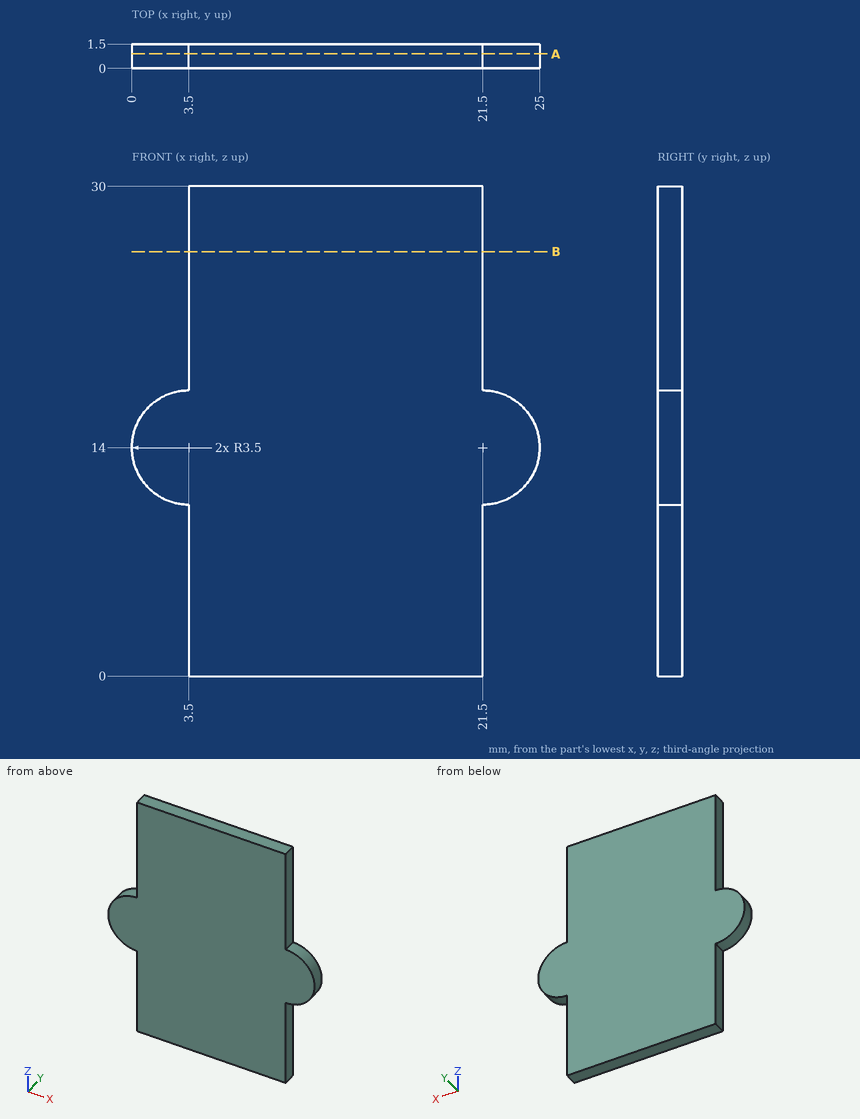
Geometry: see drawing. Coordinates: mm, zero at the bounding-box minimum. Round coordinates to 2 decimals unless told otherwise and drop trailing zeros. Write each loop counter-clockwise with the first axis right and the second up, starting at its lowest first coordinate (ties: lowest second). Pieces come first, ordered by that corner, then holes.
1) Cut plane B-B (z = 26). Return the cut outline in (x, y), then the cut area to 3 significant figures.
2) Contact query for a flat-ended pin moving along its axis: P1, Ø5, axis at x = 22.5, z = 22.5, coming from the -Y side. Output: stop coordinate, or through.
3) Cut plane A-A (y = 0.9). Return the cut outline in (x, z).
4) Ray query, L1, parallel to X at y = 1, z = 17.75; L2, parallel to X at y = 0.55, z = 11; L3, parallel to Z at x = 1, y = 1. Return the intervals inside material, ascending.
Geometry says:
1. outline: (3.5, 0) - (21.5, 0) - (21.5, 1.5) - (3.5, 1.5) - close
1. area: 27.0 mm2
2. P1: stops at y = 0
3. outline: (3.5, 0) - (21.5, 0) - (21.5, 10.5) arc R3.5 ccw to (21.5, 17.5) - (21.5, 30) - (3.5, 30) - (3.5, 17.5) arc R3.5 ccw to (3.5, 10.5) - close
4. L1: x = 3.5 to 21.5
4. L2: x = 1.7 to 23.3
4. L3: z = 11.55 to 16.45
